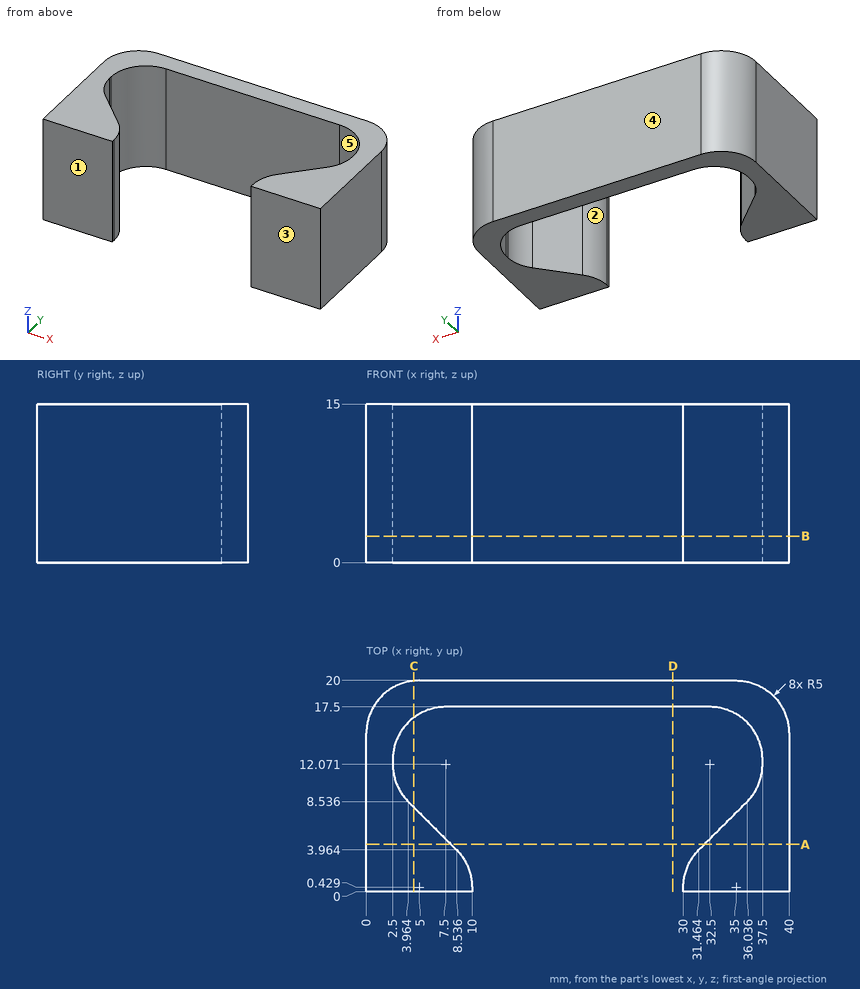
The figure shows three views and two pictorial views of one solid part (mm, origin at its lowest corner). Answer the questions. A direction names the side the tool comes from. Give positions to 0.01 mm unless a question says otherwise; leave off trailing zeros. Loops run counter-clockwise (first coordinate to the right, second up) from the corner with the lowest first, then second, coordinate; pieces in that order, holes last. Notation, with made-up numbers: (-33.75, 65.25) -> (-0.75, 65.25) arc R6 cw to (-0.75, 73.25) -> close; hole circle Ø9 at (75.5, 77). An arc over 180 degrees is marked (long way). Use a Markdown table: item, result. Add a question column.
1. Find the intervals of material crossed by probe 1 along Y at (x, z) = (26, 1); probe 2 along X at (y, z) = (7.75, 11.5); probe 3 along Y at (x, z) = (37, 12.5) (1 decimal), in increasing order.
2. Section A-A on y = 4.5 is taken. Determine the outline of the cut face in (x, z), and give its area (3 significant figures).
3. Determine the mould class of the marked faces 3, 4 and 5 for opening direction Y: released by +Y, released by -Y, zero draft, split by the parting line, or undercut.
4. For the marked faces 1 and 2, determine the directions among +Z, -Z, +X, -X, +Y, -Y from which every point of the face is accessible in a straight line to the end or side of a thin tool.
5. Section C-C on x = 4.5 is taken. Determine the outline of the cut face in (y, z) (1 decimal), and give its area (3 significant figures).
6. A flat-ended cylindrical pin translates along its axis: pin 1 Ø1 at (x, z) = (17, 2) entering from -Y. Find the tip coordinate at first contact, or state that the pin passes through.
7. Section D-D on x = 29 is taken. Determine the outline of the cut face in (y, z), and give its area (3 significant figures).
8. Section B-B on z = 2.5 is taken. Determine the outline of the cut face in (x, y) (1 decimal).
Results below:
| question | item | result |
|---|---|---|
| 1 | probe 1 | y = 17.5 to 20 |
| 1 | probe 2 | x = 0 to 4.75, 35.25 to 40 |
| 1 | probe 3 | y = 0 to 9.9, 14.7 to 19.6 |
| 2 | outline | (0, 0) -> (8, 0) -> (8, 15) -> (0, 15) -> close; (32, 0) -> (40, 0) -> (40, 15) -> (32, 15) -> close |
| 2 | area | 240 mm^2 |
| 3 | face 3 | released by -Y |
| 3 | face 4 | released by +Y |
| 3 | face 5 | undercut |
| 4 | face 1 | +Z, -Z, +X, -X, -Y |
| 4 | face 2 | +Z, -Z |
| 5 | outline | (0, 0) -> (8, 0) -> (8, 15) -> (0, 15) -> close; (16.5, 0) -> (20, 0) -> (20, 15) -> (16.5, 15) -> close |
| 5 | area | 172 mm^2 |
| 6 | pin 1 | stops at y = 17.5 |
| 7 | outline | (17.5, 0) -> (20, 0) -> (20, 15) -> (17.5, 15) -> close |
| 7 | area | 37.5 mm^2 |
| 8 | outline | (0, 0) -> (10, 0) -> (10, 0.4) arc R5 ccw to (8.5, 4) -> (4, 8.5) arc R5 cw to (2.5, 12.1) -> (2.5, 12.5) arc R5 cw to (7.5, 17.5) -> (32.5, 17.5) arc R5 cw to (37.5, 12.5) -> (37.5, 12.1) arc R5 cw to (36, 8.5) -> (31.5, 4) arc R5 ccw to (30, 0.4) -> (30, 0) -> (40, 0) -> (40, 15) arc R5 ccw to (35, 20) -> (5, 20) arc R5 ccw to (0, 15) -> close |
